from build123d import *

# Parameters (mm, degrees)
BOSS_EXTRUDE1_DEPTH         = 3
SKETCH2_W                   = 15
SKETCH2_H                   = 5
DESTEK_BAGLANT_DEPTH        = 4
SKETCH5_R                   = 5
SKETCH5_R_2                 = 1.25
MOTOR_DEPTH                 = 4
CUT_EXTRUDE2_DEPTH          = 4
CUT_EXTRUDE3_DEPTH          = 4
BOSS_EXTRUDE2_DEPTH         = 3
SKETCH9_W                   = 15.2
SKETCH9_H                   = 5.2
DESTEK_BAGLANTI_OFSET_DEPTH = 4


with BuildPart() as part:
    # Sketch1 → Boss-Extrude1 (new body)
    with BuildSketch(Plane(origin=(0, 0, 0), x_dir=(1, 0, 0), z_dir=(0, 1, 0))):
        Polygon((-107, -50), (-131.748737342, -25.251262658), (-131.748737342, 50.617257402), (-117.606601718, 64.759393026), (-117.606601718, 116.580359723), (96.393398282, 116.580359723), (131.748737342, 81.225020664), (131.748737342, -25.251262658), (107, -50), align=None)
    extrude(amount=BOSS_EXTRUDE1_DEPTH)

    # Sketch2 → Destek Baglantı (cut, through all)
    with BuildSketch(Plane(origin=(0, 3, 0), x_dir=(1, 0, 0), z_dir=(0, 1, 0))):
        with Locations((80, -42.5)):
            Rectangle(SKETCH2_W, SKETCH2_H)
        with Locations((0, -42.5)):
            Rectangle(SKETCH2_W, SKETCH2_H)
        with Locations((-80, -42.5)):
            Rectangle(SKETCH2_W, SKETCH2_H)
    extrude(amount=-DESTEK_BAGLANT_DEPTH, mode=Mode.SUBTRACT)

    # Sketch5 → Motor (cut, through all)
    with BuildSketch(Plane.XZ):
        with Locations((-17.014102848, -77.239948703)):
            Circle(SKETCH5_R)
        with Locations((25.969420718, -91.474858406)):
            Circle(SKETCH5_R_2)
        with Locations((17.969420718, -91.474858406)):
            Circle(SKETCH5_R_2)
        with Locations((9.969420718, -91.474858406)):
            Circle(SKETCH5_R_2)
        with Locations((1.969420718, -91.474858406)):
            Circle(SKETCH5_R_2)
        with Locations((-3.280579282, -85.974858406)):
            Circle(SKETCH5_R_2)
        with Locations((-3.280579282, -69.974858406)):
            Circle(SKETCH5_R_2)
        with Locations((1.969420718, -64.474858406)):
            Circle(SKETCH5_R_2)
        with Locations((9.969420718, -64.474858406)):
            Circle(SKETCH5_R_2)
        with Locations((17.969420718, -64.474858406)):
            Circle(SKETCH5_R_2)
        with Locations((25.969420718, -64.474858406)):
            Circle(SKETCH5_R_2)
        with BuildLine():
            Line((24.769420718, -88.774858406), (-0.580579282, -88.774858406))
            Line((-0.580579282, -88.774858406), (-0.580579282, -67.174858406))
            Line((-0.580579282, -67.174858406), (24.769420718, -67.174858406))
            Line((24.769420718, -67.174858406), (24.769420718, -68.654987163))
            ThreePointArc((24.769420718, -68.654987163), (44.969420718, -77.974858406), (24.769420718, -87.29472965))
            Line((24.769420718, -87.29472965), (24.769420718, -88.774858406))
        make_face()
    extrude(amount=-MOTOR_DEPTH, mode=Mode.SUBTRACT)

    # Sketch6 → Cut-Extrude2 (cut, through all)
    with BuildSketch(Plane(origin=(0, 3, 0), x_dir=(1, 0, 0), z_dir=(0, 1, 0))):
        Polygon((-125.738329701, 56.627665042), (-97.454058454, 28.343393795), (-17.454058454, 28.343393795), (-17.454058454, 31.343393795), (-96.211417767, 31.343393795), (-123.617009358, 58.748985386), align=None)
    extrude(amount=-CUT_EXTRUDE2_DEPTH, mode=Mode.SUBTRACT)

    # Sketch7 → Cut-Extrude3 (cut, through all)
    with BuildSketch(Plane(origin=(0, 3, 0), x_dir=(1, 0, 0), z_dir=(0, 1, 0))):
        Polygon((-95, -32), (95, -32), (97, -30), (-97, -30), align=None)
        Polygon((-100, -27), (-102, -25), (102, -25), (100, -27), align=None)
    extrude(amount=-CUT_EXTRUDE3_DEPTH, mode=Mode.SUBTRACT)

    # Sketch8 → Boss-Extrude2 (add, through all)
    with BuildSketch(Plane(origin=(0, 3, 0), x_dir=(1, 0, 0), z_dir=(0, 1, 0))):
        Polygon((-17.454058454, 31.343393795), (-17.454058454, 28.343393795), (-20.454058454, 28.343393795), align=None)
    extrude(amount=-BOSS_EXTRUDE2_DEPTH)

    # Sketch9 → Destek Baglanti Ofset (cut, through all)
    with BuildSketch(Plane(origin=(0, 3, 0), x_dir=(1, 0, 0), z_dir=(0, 1, 0))):
        with Locations((-80, -42.5)):
            Rectangle(SKETCH9_W, SKETCH9_H)
        with Locations((0, -42.5)):
            Rectangle(SKETCH9_W, SKETCH9_H)
        with Locations((80, -42.5)):
            Rectangle(SKETCH9_W, SKETCH9_H)
    extrude(amount=-DESTEK_BAGLANTI_OFSET_DEPTH, mode=Mode.SUBTRACT)


solid = part.part
Part model, mm, in its own coordinate system. A direction names the side the tool comes from. Round coordinates to 2 decimals unless told otherwise and drop trailing zeros. Write each loop counter-clockwise with the first axis right and the second up, starting at its lowest first coordinate (ties: lowest second). Pieces come first, ordered by that corner, then holes. Notation, with made-up numbers: M 33,-33 L 92,-33 A9 cw 92,-18 Z; hole C 18.25,37 d10. An arc over 180 degrees is marked long. Return JSON: item names as keys, results as strings. Group by question number.
(1) Saw through at C-C on z = -47. Write the cut outline in (x, y), then the cut area to 3 significant figures.
(2) Saw through at D-D on x = -27.5. Write the cut outline in (y, z), then the cut area to 3 significant figures.
(3) Which spindle directions (+Z, -Z, +X, -X, +Y, -Y) get a long thin tool onto all of the face, cutting with end or side? Do faces 4 (the face through (-111.79, 1.52, -42.68)), 5 (the face through (-128.786, 1.479, -53.58)). Say none if no direction does.
(4) Drill centre lines: probe 1 along Z at (x, y) = (-85.5, 2.15); probe 2 along Z at (x, y) = (53.5, 1.1); probe 3 along Z at (x, y) = (-68.5, 2.8). Where is each one in solid material? Low to high.
(5) Saw through at A-A on x = 22. Write the cut outline in (y, z).
(6) Two-plate mould, pull along X, no slides. Class faces 1 (the face through (2, 3, -34)), 2 (the face through (-14.33, 1.48, -73.02)), 3 (the face through (-119, 1, 38)): +X half, -X half, draft (parallel to the pull), parting line (faces both ways), or undercut.
(7) Saw through at B-B on x = 60.5. Write the cut outline in (y, z).
(8) Pin check, flat tips, straight feed: pin 1 Ø2 at (x, z) = (25.97, -64.47) entering from -Y; pin 2 Ø1 at (y, z) = (2, -82.5) entering from +X; pin 3 Ø1 at (y, z) = (2.5, -53) entering from -X; pin 4 Ø1.5 at (y, z) = (1.5, 42) entering from -X. Stop position of each tip, or through.
Returned:
{
 "1": {"outline": "M -131.75,0 L -116.11,0 L -116.11,3 L -131.75,3 Z; M -111.87,0 L 131.75,0 L 131.75,3 L -111.87,3 Z", "area": "778 mm²"},
 "2": {"outline": "M 0,-116.58 L 3,-116.58 L 3,-31.34 L 0,-31.34 Z; M 0,-28.34 L 3,-28.34 L 3,25 L 0,25 Z; M 0,27 L 3,27 L 3,30 L 0,30 Z; M 0,32 L 3,32 L 3,50 L 0,50 Z", "area": "479 mm²"},
 "3": {"face 4": "+Y, -Y", "face 5": "-Z, -X, +Y, -Y"},
 "4": {"probe 1": "-116.58 to -31.34, -28.34 to 25, 27 to 30, 32 to 39.9, 45.1 to 50", "probe 2": "-116.58 to 25, 27 to 30, 32 to 50", "probe 3": "-116.58 to -31.34, -28.34 to 25, 27 to 30, 32 to 50"},
 "5": {"outline": "M 0,-116.58 L 3,-116.58 L 3,-88.77 L 0,-88.77 Z; M 0,-67.17 L 3,-67.17 L 3,25 L 0,25 Z; M 0,27 L 3,27 L 3,30 L 0,30 Z; M 0,32 L 3,32 L 3,50 L 0,50 Z"},
 "6": {"face 1": "draft", "face 2": "undercut", "face 3": "-X half"},
 "7": {"outline": "M 0,-116.58 L 3,-116.58 L 3,25 L 0,25 Z; M 0,27 L 3,27 L 3,30 L 0,30 Z; M 0,32 L 3,32 L 3,50 L 0,50 Z"},
 "8": {"pin 1": "through", "pin 2": "x = 130.97", "pin 3": "x = -129.87", "pin 4": "x = -115.75"}
}
